Geometry check sheet. Reference: drawing and pictorial views, mm from the part's lowest x, y, z. A direction names the side the tool comes from. Round coordinates to 2 decimals unless told otherwise and drop trailing zeros. Order: outer loops, then holes, each group sorted by start corner. A loop starts at its lowest first (then second) coordinate and runs counter-clockwise, first axis right, second up.
(1) Sectioned sample at D-D, the plane x = 7.5. Enter the section's corners in (y, z), and give its area (3 significant figures).
(2) Tool access check on the marked faces 1, 2 and 3. Record the directions out of +Z, -Z, +X, -X, +Y, -Y that give a thin tool (end or side, any length) a straight path to the whole face; none if there is none.
(3) Thickness scan on probe 1 along Y at (x, z) = (30.5, 4.25); probe 2 along X at (y, z) = (92.5, 7); probe 3 along X at (y, z) = (25, 2). Record the ranges inside material, lowest first.
(4) Sectioned sample at A-A, the plane x = 26. Enter the section's corners in (y, z).
(5) Sectioned sample at C-C, the plane y = 82. Enter the section's corners in (x, z), and give its area (3 significant figures).
(6) Depth check by flat-ended pin: pin 1 (4 mm diameter, centred on x = 7.5, z = 2, fed in from -Y); pin 2 (1.1 mm diameter, centred on x = 33, z = 6.5, fed in from -Y); pin 3 (6 mm diameter, centred on x = 46, z = 5, fed in from +Y); pin 4 (3.5 mm diameter, centred on x = 26.5, z = 6, fed in from -Y). Enter the tip coordinate at first touch or a pass-through.
(7) Sectioned sample at B-B, the plane z = 6.25. Enter the section's corners in (x, y).
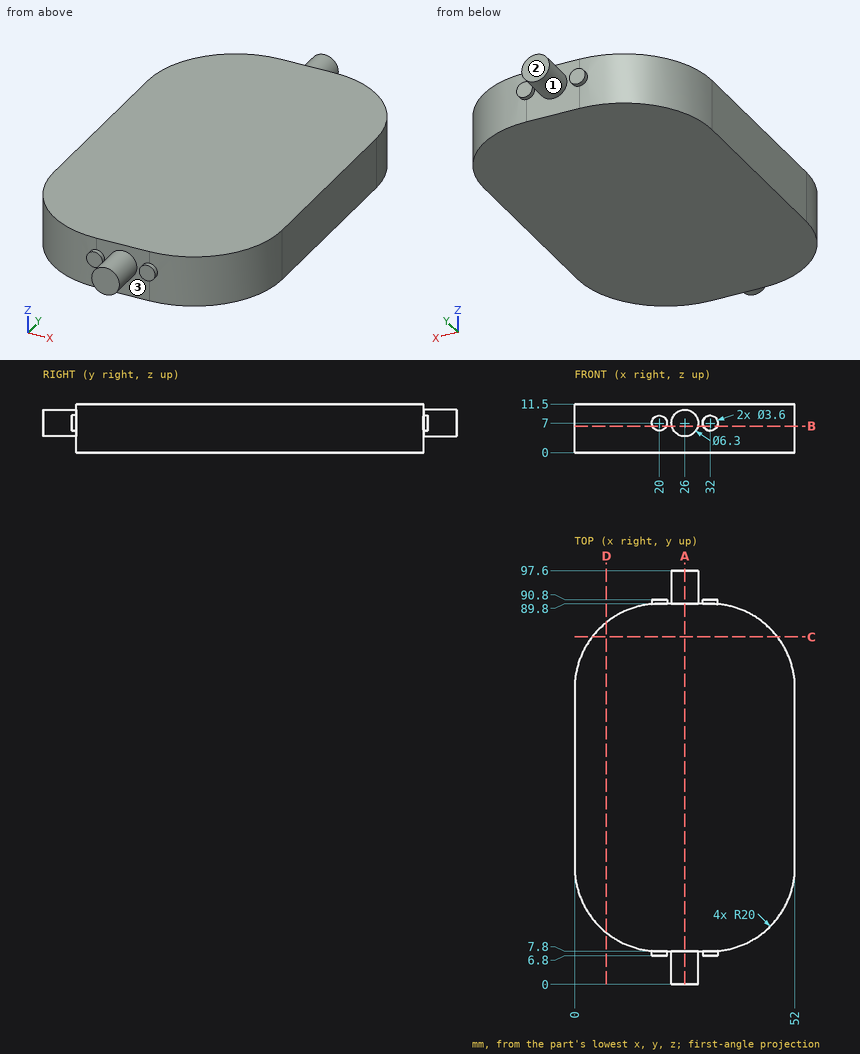
Derived:
1. outline: (12.19, 0) - (85.41, 0) - (85.41, 11.5) - (12.19, 11.5) - close
1. area: 842 mm2
2. face 1: +Y
2. face 2: +Z, -Z, +X, -X, +Y
2. face 3: -Y
3. probe 1: y = 7.8 to 89.8
3. probe 2: x = 22.85 to 29.15
3. probe 3: x = 0.2 to 51.8
4. outline: (0, 3.85) - (7.8, 3.85) - (7.8, 0) - (89.8, 0) - (89.8, 3.85) - (97.6, 3.85) - (97.6, 10.15) - (89.8, 10.15) - (89.8, 11.5) - (7.8, 11.5) - (7.8, 10.15) - (0, 10.15) - close
5. outline: (4.15, 0) - (47.85, 0) - (47.85, 11.5) - (4.15, 11.5) - close
5. area: 503 mm2
6. pin 1: stops at y = 10.78
6. pin 2: stops at y = 6.8
6. pin 3: stops at y = 86.5
6. pin 4: stops at y = 0
7. outline: (0, 27.8) arc R20 ccw to (18.36, 7.87) - (18.36, 6.8) - (21.64, 6.8) - (21.64, 7.8) - (22.94, 7.8) - (22.94, 0) - (29.06, 0) - (29.06, 7.8) - (30.36, 7.8) - (30.36, 6.8) - (33.64, 6.8) - (33.64, 7.87) arc R20 ccw to (52, 27.8) - (52, 69.8) arc R20 ccw to (33.64, 89.73) - (33.64, 90.8) - (30.36, 90.8) - (30.36, 89.8) - (29.06, 89.8) - (29.06, 97.6) - (22.94, 97.6) - (22.94, 89.8) - (21.64, 89.8) - (21.64, 90.8) - (18.36, 90.8) - (18.36, 89.73) arc R20 ccw to (0, 69.8) - close
